```python
from build123d import *

# Parameters (mm, degrees)
PAD_DEPTH         = 3.9
PAD_DEPTH_BACK    = 2.3
POCKET_DEPTH      = 0.01
POCKET_DEPTH_BACK = 20
POCKET001_DEPTH   = 1.35
PAD001_DEPTH      = 12
POCKET002_DEPTH   = 5
SKETCH004_W       = 5
SKETCH004_H       = 4
POCKET003_DEPTH   = 5
SKETCH006_W       = 4.5
SKETCH006_H       = 5.5
SKETCH006_W_2     = 3.7
SKETCH006_H_2     = 2.7
POCKET004_DEPTH   = 5
PRISM_DEPTH       = 3
PRISM001_DEPTH    = 3


with BuildPart() as part:
    # Sketch → Pad (new body, two sides)
    with BuildSketch(Plane.XY) as pad_sk:
        with BuildLine():
            Line((-0.86, -0.86), (19.26, -0.86))
            Line((19.26, -0.86), (19.26, 25.7000002895))
            ThreePointArc((19.26, 25.7000002895), (9.1999999842, 35.7600003468), (-0.86, 25.7000002578))
            Line((-0.86, -0.86), (-0.86, 25.7000002578))
        make_face()
    extrude(amount=PAD_DEPTH)
    extrude(pad_sk.sketch, amount=-PAD_DEPTH_BACK)

    # Sketch001 → Pocket (cut, two sides)
    with BuildSketch(Plane.XY) as pocket_sk:
        with BuildLine():
            Line((1e-10, 25.6999686791), (1e-10, 0))
            Line((1e-10, 0), (18.4, 0))
            Line((18.4, 0), (18.4, 25.7))
            ThreePointArc((18.4, 25.7), (9.1999843395, 34.9), (1e-10, 25.6999686791))
        make_face()
    extrude(amount=-POCKET_DEPTH, mode=Mode.SUBTRACT)
    extrude(pocket_sk.sketch, amount=POCKET_DEPTH_BACK, mode=Mode.SUBTRACT)

    # Sketch003 → Pocket001 (cut)
    with BuildSketch(Plane.XY):
        with BuildLine():
            Line((17.4, 10), (13.4, 10))
            Line((13.4, 10), (13.4, 0))
            Line((13.4, 0), (0.8, 0))
            Line((0.8, 0), (0.8, 4))
            Line((0.8, 4), (0, 4))
            Line((0, 4), (0, 17))
            Line((0, 17), (2, 17))
            Line((2, 17), (2, 21))
            Line((2, 21), (0, 21))
            Line((1e-10, 25.6999686791), (0, 21))
            ThreePointArc((2.0291307695, 31.4635609201), (0.5220919157, 28.7551450506), (1e-10, 25.6999686791))
            Line((2.0291307695, 31.4635609201), (6.4, 31.4635609201))
            Line((6.4, 31.4635609201), (6.4, 34.4635609201))
            ThreePointArc((10.2, 34.8454906921), (8.2799632683, 34.8538807296), (6.4, 34.4635609201))
            Line((10.2, 34.8454906921), (10.2, 32.4454906921))
            Line((10.2, 32.4454906921), (15.4560654826, 32.4454906921))
            ThreePointArc((18.4, 25.7), (17.6319571405, 29.3799590732), (15.4560654826, 32.4454906921))
            Line((18.4, 25.7), (18.4, 17))
            Line((15.4, 17), (18.4, 17))
            Line((15.4, 15.5), (15.4, 17))
            Line((18.4, 15.5), (15.4, 15.5))
            Line((18.4, 15.5), (18.4, 2))
            Line((17.4, 2), (18.4, 2))
            Line((17.4, 10), (17.4, 2))
        make_face()
    extrude(amount=-POCKET001_DEPTH, mode=Mode.SUBTRACT)

    # Sketch007 (on Face8 of Pocket001) → Pad001 (join)
    with BuildSketch(Plane(origin=(0, 8, 0), x_dir=(-1, 0, 0), z_dir=(0, 1, 0))):
        Polygon((-1e-10, 0.79), (-0.2000000001, 0.99), (-0.2000000001, 1.39), (-1e-10, 1.59), align=None)
        Polygon((-18.4, 1.59), (-18.2, 1.39), (-18.2, 0.99), (-18.4, 0.79), align=None)
    extrude(amount=PAD001_DEPTH)

    # Sketch002 (on Face2 of Pocket) → Pocket002 (cut)
    with BuildSketch(Plane(origin=(-0.86, 0, 0), x_dir=(0, -1, 0), z_dir=(-1, 0, 0))):
        Polygon((-18.2, -0.01), (-18.2, 3.99), (-9.3, 3.99), (-9.3, -0.01), (-12, -0.01), (-12, -1.19), (-15, -1.19), (-15, -0.01), align=None)
    extrude(amount=-POCKET002_DEPTH, mode=Mode.SUBTRACT)

    # Sketch004 (on Face3 of Pocket002) → Pocket003 (cut)
    with BuildSketch(Plane.YZ.offset(19.26)):
        with Locations((15, 2)):
            Rectangle(SKETCH004_W, SKETCH004_H)
    extrude(amount=-POCKET003_DEPTH, mode=Mode.SUBTRACT)

    # Sketch006 (on Face4 of Pocket003) → Pocket004 (cut)
    with BuildSketch(Plane(origin=(0, 0, -2.3), x_dir=(1, 0, 0), z_dir=(0, 0, -1))):
        with Locations((2.75, -7.75)):
            Rectangle(SKETCH006_W, SKETCH006_H)
        with Locations((11.55, -16.65)):
            Rectangle(SKETCH006_W_2, SKETCH006_H_2)
    extrude(amount=-POCKET004_DEPTH, mode=Mode.SUBTRACT)

    # Prism → Prism (cut)
    with BuildSketch(Plane(origin=(7.49996936, 34.6999942124, 2.9), x_dir=(3.4044e-06, -1, 0), z_dir=(1, 3.4044e-06, 0))):
        Polygon((0.4, 0), (0.2, 0.3464101615), (-0.2, 0.3464101615), (-0.4, 0), (-0.2, -0.3464101615), (0.2, -0.3464101615), align=None)
    extrude(amount=PRISM_DEPTH, mode=Mode.SUBTRACT)

    # Prism001 → Prism001 (cut)
    with BuildSketch(Plane(origin=(7.5000000001, 0, 2.9), x_dir=(0, -1, 0), z_dir=(1, 0, 0))):
        Polygon((0.4, 0), (0.2, 0.3464101615), (-0.2, 0.3464101615), (-0.4, 0), (-0.2, -0.3464101615), (0.2, -0.3464101615), align=None)
    extrude(amount=PRISM001_DEPTH, mode=Mode.SUBTRACT)


solid = part.part
```
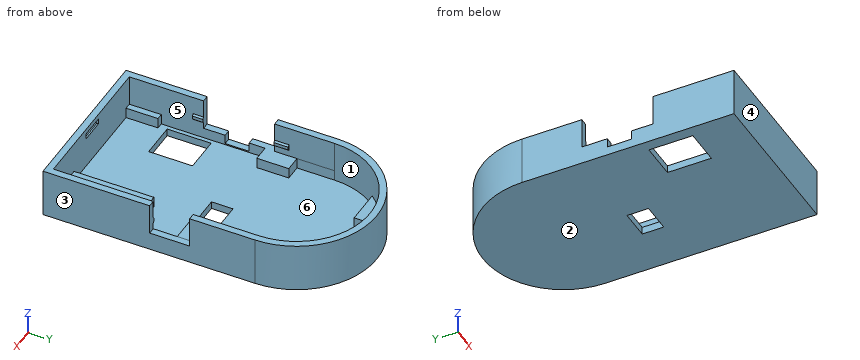
Work out the finished part from the listing and answer in its coordinate system (mm). Face numbers are marked on the shaded views. A direction names the side the tool comes from. Coordinates: 2 decimals unless noted, no trailing zeros. Loops run counter-clockwise (first coordinate to the right, second up) from the corner with the lowest first, then second, coordinate; pieces in that order, holes last. Notation, with made-up numbers: (74.5, 15) - (95.5, 15) arc R29 ccw to (95.5, 38) - close; hole circle Ø9 at (20.25, 11.5). An arc over 180 degrees is marked (long way). Use a Markdown table: item, result.
Item 1: Find section D-D, the plane y = 30.5. Determine the outline of the cut face in (x, z).
Evaluation:
| item | result |
|---|---|
| outline | (0.36, -2.3) - (18.04, -2.3) - (18.04, 3.9) - (17.05, 3.9) - (17.05, -1.35) - (1.35, -1.35) - (1.35, 3.9) - (0.36, 3.9) - close |
Item 2: For the marked faces 1 and 2, determine the directions among +Z, -Z, +X, -X, +Y, -Y from which every point of the face is accessible in a straight line to the end or side of a thin tool.
Evaluation:
| item | result |
|---|---|
| face 1 | +Z |
| face 2 | -Z, +X, -X, +Y, -Y |
Item 3: The mould has two halves that part along Y. Classify the marked faces 3, 4, 5 and 6: +Y half, -Y half, draft (parallel to the pull), parting line (faces both ways), or undercut.
Evaluation:
| item | result |
|---|---|
| face 3 | draft |
| face 4 | -Y half |
| face 5 | undercut |
| face 6 | undercut |
Item 4: Given pin 1 Ø5 at (x, y) = (7.5, 15.5) entering from +Z; pin 2 Ø0.6 at (x, y) = (0.5, 1.5) entering from +Z; pin 3 Ø0.7 at (x, z) = (1, -0.5) entering from +Y, each flat-ended and moving along its own axis, determine where each tip first touches the part or whether it passes through.
Evaluation:
| item | result |
|---|---|
| pin 1 | stops at z = -1.35 |
| pin 2 | stops at z = -0.01 |
| pin 3 | stops at y = 31.99 |
Item 5: Consider probe 1 along X at (y, z) = (6, 2.25); probe 2 along X at (y, z) = (20, -0.5); probe 3 along Y at (x, z) = (16.5, -0.5). Determine where each line is inside the solid, lowest interval first. Write a range as from..to.
Evaluation:
| item | result |
|---|---|
| probe 1 | x = -0.86..0, 18.4..19.26 |
| probe 2 | x = -0.86..2, 18.4..19.26 |
| probe 3 | y = -0.86..10, 15.5..17, 31.3..32.62 |
Item 6: Find section B-B, the plane x = 12.25. Determine the outline of the cut face in (y, z).
Evaluation:
| item | result |
|---|---|
| outline | (-0.86, -2.3) - (15.3, -2.3) - (15.3, -1.35) - (0, -1.35) - (0, 3.9) - (-0.86, 3.9) - close; (18, -2.3) - (35.29, -2.3) - (35.29, 3.9) - (34.38, 3.9) - (34.38, -0.01) - (32.45, -0.01) - (32.45, -1.35) - (18, -1.35) - close |
Item 7: Find section C-C, the plane x = 14.5. Determine the outline of the cut face in (y, z), and give its area (3 significant figures).
Evaluation:
| item | result |
|---|---|
| outline | (-0.86, -2.3) - (34.25, -2.3) - (34.25, 3.9) - (33.22, 3.9) - (33.22, -0.01) - (32.45, -0.01) - (32.45, -1.35) - (10, -1.35) - (10, -0.01) - (0, -0.01) - (0, 3.9) - (-0.86, 3.9) - close |
| area | 57.7 mm2 |
Item 8: Find section A-A, the plane y = 11. Determine the outline of the cut face in (x, z).
Evaluation:
| item | result |
|---|---|
| outline | (-0.86, -2.3) - (19.26, -2.3) - (19.26, 3.9) - (18.4, 3.9) - (18.4, 1.59) - (18.2, 1.39) - (18.2, 0.99) - (18.4, 0.79) - (18.4, -1.35) - (0, -1.35) - (0, -0.01) - (-0.86, -0.01) - close |
